Part model, mm, in its own coordinate system. A direction names the side the tool comes from. Give positions to 0.01 mm unless a question says otherwise; leave off trailing zeros. Order: outer loops, then holes, each group sorted by start corner. A loop starts at its lowest first (then second) coordinate and runs counter-clockwise, first axis right, second up. Notation, with made-up numbers: (28, 46) - (72, 46) arc R10 ccw to (72, 61) - close; hole circle Ø7 at (9.25, 72.5). An arc over 180 degrees is marked (long way). Use one line per item in the form item = value. Start each with the question number.
1. Band-saw the part on A-A, the plane z = 8.75. List the corners of the cut face in (x, y).
2. Band-saw the part on B-B, the plane x = 36. State how many separate pieces and enclosed holes the cut face has, plus the area to 3 significant figures.
3. Band-saw the part on D-D, the plane z = 18. List the corners of the cut face in (x, y), plus the area to 3 significant figures.
4. Pin check, flat tips, straight feed: P1, Ø2, axis at y = -17, z = 13, coming from the +X side; P2, Ø1.5, axis at y = -11.5, z = 11, coming from the +X side; P3, Ø1, axis at y = -15.5, z = 5.5, coming from the -X side; P4, Ø4, axis at x = 36, y = -36, coming from the -Z side. Stop position of each tip, or through.
5. Pull direction X, two halves, no side cores. Call faces 4 (the face through (30, 30, 3.8)), 5 (the face through (37.21, -34.103, 1.873)), 6 (the face through (-40, -1, 2)): +X half, -X half, draft (parallel to the pull), parting line (faces both ways), or undercut.
6. Tool access for faces 1 (the face through (-39.05, 8.67, 4.19)), 2 (the face through (-4.88, 37.18, 1.87)), 3 (the face through (30, -32, 3.8)): list every direction of +Z, -Z, +X, -X, +Y, -Y with a clear straight run to the whole face (end or side of a thin tool).
7. Drill centre lines: line 1 (X direction, y = 0, z = 2.3); line 2 (Y direction, x = -22.5, z = 3.75); line 3 (X direction, y = 4, z = 13.75). Where is each one in solid material? Low to high.
from build123d import *

# Parameters (mm, degrees)
F0_W     = 80
F0_H     = 80
F0_R     = 2.25
F0_R_2   = 37.5
F1_DEPTH = 3.8


# Not quite as in the source:
# - a feature names something its author has since deleted; it is built from what else it names


with BuildPart() as f1:
    # F0 (on Top) → F1 (new body)
    with BuildSketch(Plane.XY):
        Rectangle(F0_W, F0_H)
        with Locations((-36, -36)):
            Circle(F0_R, mode=Mode.SUBTRACT)
        with Locations((36, -36)):
            Circle(F0_R, mode=Mode.SUBTRACT)
        with Locations((-36, 36)):
            Circle(F0_R, mode=Mode.SUBTRACT)
        Circle(F0_R_2, mode=Mode.SUBTRACT)
        with Locations((36, 36)):
            Circle(F0_R, mode=Mode.SUBTRACT)
    extrude(amount=F1_DEPTH)

    # F2 (on Right) → F3 (revolve)
    with BuildSketch(Plane.YZ):
        Polygon((-40, 0), (-37.5, 0), (-37.5, 3.8), (-13.5, 20.2198829502), (-13.5, 22.7198829502), (-40, 4.589595526), (-40, 3.8), align=None)
    revolve(axis=Axis((0, 0, 27.8761722147), (0, 0, 1)))


solid = f1.part
From the geometry:
q1.outline = circle Ø67.84 at (0, 0); hole circle Ø60.53 at (0, 0)
q2.separate_pieces = 3
q2.enclosed_holes = 0
q2.area = 266 mm²
q3.outline = circle Ø40.8 at (0, 0); hole circle Ø33.49 at (0, 0)
q3.area = 426 mm²
q4.P1 = 23.84
q4.P2 = 29.6
q4.P3 = -36.25
q4.P4 = through
q5.face_4 = draft
q5.face_5 = undercut
q5.face_6 = -X half
q6.face_1 = +Z
q6.face_2 = -Z
q6.face_3 = +Z, +X, -Y
q7.line_1 = -40 to -37.5, 37.5 to 40
q7.line_2 = -40 to -30, 30 to 40
q7.line_3 = -26.31 to -22.61, 22.61 to 26.31
